```python
from build123d import *

# Parameters (mm, degrees)
ESQUISSE1_W               = 70
ESQUISSE1_H               = 55
ESQUISSE1_R               = 9
BOSS_EXTRU_1_DEPTH        = 4
ESQUISSE2_R               = 11
ENL_V_MAT_EXTRU_1_DEPTH   = 5.5
TROU_TARAUD_M4X0_71_D     = 3
TROU_TARAUD_M4X0_71_DEPTH = 15
TROU_TARAUD_M4X0_71_TIP   = 0.901290929
TROU_TARAUD_M4X0_72_D     = 3
TROU_TARAUD_M4X0_72_DEPTH = 15
TROU_TARAUD_M4X0_72_TIP   = 0.901290929
TROU_TARAUD_M4X0_73_D     = 3
TROU_TARAUD_M4X0_73_DEPTH = 15
TROU_TARAUD_M4X0_73_TIP   = 0.901290929
TROU_TARAUD_M4X0_74_D     = 3
TROU_TARAUD_M4X0_74_DEPTH = 15
TROU_TARAUD_M4X0_74_TIP   = 0.901290929
BOSS_EXTRU_2_START        = 7
ESQUISSE11_R              = 17.5
ESQUISSE11_R_2            = 11
BOSS_EXTRU_2_DEPTH        = 7


with BuildPart() as part:
    # Esquisse1 → Boss.-Extru.1 (new, symmetric)
    with BuildSketch(Plane(origin=(0, 0, 0), x_dir=(0, 0, -1), z_dir=(1, 0, 0))):
        with Locations((0, 7.5)):
            Rectangle(ESQUISSE1_W, ESQUISSE1_H)
        Circle(ESQUISSE1_R, mode=Mode.SUBTRACT)
    extrude(amount=BOSS_EXTRU_1_DEPTH, both=True)

    # Esquisse2 → Enlèv. mat.-Extru.1 (cut)
    with BuildSketch(Plane(origin=(4, 0, 0), x_dir=(0, 0, -1), z_dir=(1, 0, 0))):
        Circle(ESQUISSE2_R)
    extrude(amount=-ENL_V_MAT_EXTRU_1_DEPTH, mode=Mode.SUBTRACT)

    # Trou taraudé M4x0.71
    with Locations(Plane(origin=(0, -20, 0), x_dir=(-1, 0, 0), z_dir=(0, -1, 0))):
        with Locations((0, -25), (0, 25)):
            Hole(TROU_TARAUD_M4X0_71_D / 2, depth=TROU_TARAUD_M4X0_71_DEPTH)
            with Locations((0, 0, -(TROU_TARAUD_M4X0_71_DEPTH + TROU_TARAUD_M4X0_71_TIP / 2))):  # 118° drill point
                Cone(0, TROU_TARAUD_M4X0_71_D / 2, TROU_TARAUD_M4X0_71_TIP, mode=Mode.SUBTRACT)

    # Trou taraudé M4x0.72
    with Locations(Plane(origin=(0, 35, 0), x_dir=(1, 0, 0), z_dir=(0, 1, 0))):
        with Locations((0, -25), (0, 25)):
            Hole(TROU_TARAUD_M4X0_72_D / 2, depth=TROU_TARAUD_M4X0_72_DEPTH)
            with Locations((0, 0, -(TROU_TARAUD_M4X0_72_DEPTH + TROU_TARAUD_M4X0_72_TIP / 2))):  # 118° drill point
                Cone(0, TROU_TARAUD_M4X0_72_D / 2, TROU_TARAUD_M4X0_72_TIP, mode=Mode.SUBTRACT)

    # Trou taraudé M4x0.73
    with Locations(Plane.XY.offset(35)):
        with Locations((0, 7.5)):
            Hole(TROU_TARAUD_M4X0_73_D / 2, depth=TROU_TARAUD_M4X0_73_DEPTH)
            with Locations((0, 0, -(TROU_TARAUD_M4X0_73_DEPTH + TROU_TARAUD_M4X0_73_TIP / 2))):  # 118° drill point
                Cone(0, TROU_TARAUD_M4X0_73_D / 2, TROU_TARAUD_M4X0_73_TIP, mode=Mode.SUBTRACT)

    # Trou taraudé M4x0.74
    with Locations(Plane(origin=(0, 0, -35), x_dir=(-1, 0, 0), z_dir=(0, 0, -1))):
        with Locations((0, 7.5)):
            Hole(TROU_TARAUD_M4X0_74_D / 2, depth=TROU_TARAUD_M4X0_74_DEPTH)
            with Locations((0, 0, -(TROU_TARAUD_M4X0_74_DEPTH + TROU_TARAUD_M4X0_74_TIP / 2))):  # 118° drill point
                Cone(0, TROU_TARAUD_M4X0_74_D / 2, TROU_TARAUD_M4X0_74_TIP, mode=Mode.SUBTRACT)

    # Esquisse11 → Boss.-Extru.2 (add)
    with BuildSketch(Plane(origin=(-1.5, 0, 0), x_dir=(0, 0, -1), z_dir=(1, 0, 0)).offset(BOSS_EXTRU_2_START)):
        with Locations(Location((0, 0, 0), (0, 0, 180))):
            Circle(ESQUISSE11_R)
        Circle(ESQUISSE11_R_2, mode=Mode.SUBTRACT)
    extrude(amount=-BOSS_EXTRU_2_DEPTH)


solid = part.part
```
For this review, take the finished solid that the model builds, in its own axes (mm). A direction names the side the tool comes from. Coordinates: 2 decimals unless noted, no trailing zeros. Loops run counter-clockwise (first coordinate to the right, second up) from the corner with the lowest first, then second, coordinate; pieces in that order, holes last. Notation, with made-up numbers: (33, 73.5) -> (86, 73.5) arc R25 ccw to (86, 106.5) -> close; hole circle Ø8 at (73, 30.5). An arc over 180 degrees is marked (long way). Return JSON: item names as keys, results as strings. Group by question number.
(1) For pin 1 Ø6.5 at (y, z) = (-1, 2.5) entering from +X; pin 2 Ø2.5 at (x, z) = (0, -25) entering from -Y; pin 3 Ø2.5 at (x, y) = (0, 7.5) entering from -Z; pin 4 Ø1.5 at (y, z) = (-7.5, -19) entering from +X, all flat-tipped, find the tip position at first contact; note any pin that passes through.
(2) Tool access review of faces 1 (the cylindrical face through (-0.195, -12.395, 23.513)), 2 (the cylindrical face through (0, 6, -27)), 3 (the cylindrical face through (0.195, 27.395, 23.513)): name each direction out of +Z, -Z, +X, -X, +Y, -Y from which nothing blocks a thin tool from reaching the whole face with its end or side.
(3) To check wall thickness, follow L1, parallel to Z at x = 0, y = -13.25; L2, parallel to Y at x = -3.3, z = 0; L3, parallel to Z at x = 0, y = -9.75. State the ranges of each line that lie inside material, in increasing order.
(4) Consider section B-B, the plane z = -22. Give the boundary of the cut face in (x, y), plus the area to 3 significant figures.
(5) Consider section C-C, the plane y = -6. Give the boundary of the cut face in (x, z), plus the area to 3 significant figures.
(6) Consider section D-D, the plane z = -8. Give the boundary of the cut face in (x, y).
(7) Mouldability with a two-part tool opening along Y and no side actions: class faces 4 (the flat face through (0, 35, 0)), 5 (the flat face through (-1.5, -9, -2)), 6 (the cylindrical face through (-2.768, 8.923, 1.172)), 7 (the flat face through (2, 7, -35)) as pulls with the +Y half, pulls with the -Y half, needs draft (parallel to the pull), parting line crosses it, or undercut.
(8) Consider section A-A, the plane y = 27. Give the boundary of the cut face in (x, z).
Results below:
{
 "1": {"pin 1": "passes through", "pin 2": "stops at y = -4.85", "pin 3": "stops at z = -19.85", "pin 4": "stops at x = 4"},
 "2": {"face 1": "-Y", "face 2": "-Z", "face 3": "+Y"},
 "3": {"L1": "z = -35 to -26.5, -23.5 to 23.5, 26.5 to 35", "L2": "y = -20 to -9, 9 to 35", "L3": "z = -35 to -26.5, -23.5 to -5.09, 5.09 to 23.5, 26.5 to 35"},
 "4": {"outline": "(-4, -20) -> (4, -20) -> (4, 35) -> (-4, 35) -> close; hole circle Ø3 at (0, 7.5)", "area": "433 mm2"},
 "5": {"outline": "(-4, -35) -> (4, -35) -> (4, -16.44) -> (5.5, -16.44) -> (5.5, -9.22) -> (-1.5, -9.22) -> (-1.5, -6.71) -> (-4, -6.71) -> close; (-4, 6.71) -> (-1.5, 6.71) -> (-1.5, 9.22) -> (5.5, 9.22) -> (5.5, 16.44) -> (4, 16.44) -> (4, 35) -> (-4, 35) -> close; hole circle Ø3 at (0, -25); hole circle Ø3 at (0, 25)", "area": "433 mm2"},
 "6": {"outline": "(-4, -20) -> (4, -20) -> (4, -15.56) -> (5.5, -15.56) -> (5.5, -7.55) -> (-1.5, -7.55) -> (-1.5, -4.12) -> (-4, -4.12) -> close; (-4, 4.12) -> (-1.5, 4.12) -> (-1.5, 7.55) -> (5.5, 7.55) -> (5.5, 15.56) -> (4, 15.56) -> (4, 35) -> (-4, 35) -> close"},
 "7": {"face 4": "pulls with the +Y half", "face 5": "undercut", "face 6": "undercut", "face 7": "needs draft"},
 "8": {"outline": "(-4, -35) -> (4, -35) -> (4, 35) -> (-4, 35) -> close; hole circle Ø3 at (0, -25); hole circle Ø3 at (0, 25)"}
}
